from build123d import *

# Parameters (mm, degrees)
BOSS_EXTRUDE1_OUTLINE_R = 1.75
BOSS_EXTRUDE1_DEPTH     = 4
CUT_EXTRUDE1_DEPTH      = 1


# Read off the part's stored shape, not the designer's step: Boss-Extrude1
with BuildPart() as part:
    # Boss-Extrude1 outline → Boss-Extrude1 (new body)
    with BuildSketch(Plane(origin=(0, 0, 0), x_dir=(1, 0, 0), z_dir=(0, 1, 0))):
        with BuildLine():
            Line((25.086474615, -10.33744254), (36.25307775, -10.33744254))
            ThreePointArc((36.25307775, -10.33744254), (38.689776183, -5.587442326), (41.126474615, -10.33744254))
            Line((41.126474615, -10.33744254), (48.189776182, -10.33744254))
            Line((48.189776182, -10.33744254), (48.189776182, -18.81631662))
            Line((48.189776182, -18.81631662), (58.639776182, -18.81631662))
            Line((58.639776182, -18.81631662), (58.639776182, -4.977921711))
            Line((58.639776182, -4.977921711), (-21.360223818, -4.977921711))
            Line((-21.360223818, -4.977921711), (-21.360223818, -18.81631662))
            Line((-21.360223818, -18.81631662), (-10.910223818, -18.81631662))
            Line((-10.910223818, -18.81631662), (-10.910223818, -10.33744254))
            Line((-10.910223818, -10.33744254), (4.17307775, -10.33744254))
            ThreePointArc((4.17307775, -10.33744254), (6.609776182, -5.587442326), (9.046474615, -10.33744254))
            Line((9.046474615, -10.33744254), (20.21307775, -10.33744254))
            ThreePointArc((20.21307775, -10.33744254), (22.649776182, -5.587442326), (25.086474615, -10.33744254))
        make_face()
        with Locations((-16.360223818, -13.587442433)):
            Circle(BOSS_EXTRUDE1_OUTLINE_R, mode=Mode.SUBTRACT)
        with Locations((53.639776182, -13.587442433)):
            Circle(BOSS_EXTRUDE1_OUTLINE_R, mode=Mode.SUBTRACT)
    extrude(amount=BOSS_EXTRUDE1_DEPTH)

    # Sketch2 → Cut-Extrude1 (cut)
    # profile 1 of 2: a face of its own
    with BuildSketch(Plane(origin=(0, 4, 0), x_dir=(1, 0, 0), z_dir=(0, 1, 0))):
        Polygon((-16.41198232, -6.812466594), (-14.865187448, -6.812466594), (-14.865187448, -7.382338389), (-15.842110525, -7.382338389), (-15.842110525, -7.992915312), (-14.865187448, -7.992915312), (-14.865187448, -8.562787107), (-15.842110525, -8.562787107), (-15.842110525, -9.987466594), (-16.41198232, -9.987466594), align=None)
    # profile 2 of 2: a face of its own
    with BuildSketch(Plane(origin=(0, 4, 0), x_dir=(1, 0, 0), z_dir=(0, 1, 0))):
        with BuildLine():
            Line((-13.412523186, -6.731056337), (-12.907525189, -6.987371442))
            Line((-12.907525189, -6.987371442), (-13.460860525, -8.074325568))
            add(Edge.make_bspline(
                [(-13.460860525, -8.074325568), (-13.428168252, -8.075158914), (-13.363985411, -8.076794974), (-13.269480346, -8.090388716), (-13.179110672, -8.113598896), (-13.09179585, -8.144481034), (-13.008800475, -8.185943305), (-12.928789535, -8.235267944), (-12.853832504, -8.295423778), (-12.782210807, -8.362073474), (-12.717085558, -8.435911696), (-12.660512768, -8.515253227), (-12.611210579, -8.59816766), (-12.572885042, -8.686509995), (-12.541970388, -8.778815858), (-12.519664104, -8.875454234), (-12.506937745, -8.976704968), (-12.505183204, -9.045489177), (-12.504290013, -9.080505456)],
                knots=[0, 0, 0, 0, 1.013672955, 1.990085268, 2.953345895, 3.903887042, 4.856677135, 5.825509993, 6.813434118, 7.832212698, 8.85718992, 9.860832204, 10.8510077, 11.84312444, 12.841215551, 13.86684641, 14.914066156, 16, 16, 16, 16], degree=3))
            add(Edge.make_bspline(
                [(-12.504290013, -9.080505456), (-12.505127007, -9.114259025), (-12.506781387, -9.180975356), (-12.520457023, -9.278964679), (-12.54255757, -9.372979704), (-12.57414369, -9.462832672), (-12.614292202, -9.548962785), (-12.663391114, -9.631319503), (-12.721847604, -9.7092874), (-12.78815132, -9.782452193), (-12.860632718, -9.849142442), (-12.937032061, -9.908420617), (-13.017996745, -9.957386638), (-13.101996444, -9.998739592), (-13.190577642, -10.029597853), (-13.28241472, -10.052890494), (-13.378204103, -10.06633136), (-13.443223482, -10.068021564), (-13.476124948, -10.06887685)],
                knots=[0, 0, 0, 0, 1.049934834, 2.075270938, 3.072134561, 4.05064612, 5.033440221, 6.024524368, 7.028587226, 8.060776465, 9.092543989, 10.090062252, 11.064205434, 12.031961459, 12.998029633, 13.977230324, 14.976426867, 16, 16, 16, 16], degree=3))
            add(Edge.make_bspline(
                [(-13.476124948, -10.06887685), (-13.510529884, -10.068174962), (-13.578182536, -10.066794794), (-13.677175296, -10.051340548), (-13.772117873, -10.028076335), (-13.862476674, -9.994858992), (-13.948813614, -9.952563006), (-14.03011223, -9.900225978), (-14.107057351, -9.838425045), (-14.17882863, -9.768550629), (-14.243489203, -9.692012768), (-14.30116103, -9.61254654), (-14.349951471, -9.530027246), (-14.389446195, -9.444543116), (-14.420260894, -9.356366547), (-14.44170164, -9.265330188), (-14.455672265, -9.171675513), (-14.457310002, -9.108116151), (-14.458136166, -9.076053333)],
                knots=[0, 0, 0, 0, 1.063775006, 2.091769615, 3.092589432, 4.084662827, 5.064601646, 6.061867366, 7.070035304, 8.113879863, 9.156342271, 10.166834137, 11.149076039, 12.117706134, 13.076241869, 14.034148791, 15.008317125, 16, 16, 16, 16], degree=3))
            add(Edge.make_bspline(
                [(-14.458136166, -9.076053333), (-14.457699638, -9.05122443), (-14.45682415, -9.001428418), (-14.448026022, -8.926861595), (-14.434649776, -8.852099041), (-14.419144957, -8.789012031), (-14.40317966, -8.735665362), (-14.387110466, -8.690519517), (-14.367196241, -8.640417501), (-14.344431332, -8.585231374), (-14.318099865, -8.525027523), (-14.288339392, -8.45997005), (-14.255075822, -8.38956629), (-14.231354315, -8.341209808), (-14.218993538, -8.316012267)],
                knots=[0, 0, 0, 0, 1.110454016, 2.227089276, 3.35462975, 4.507227546, 5.131400587, 5.845402449, 6.650387134, 7.543487832, 8.516250726, 9.590168902, 10.744287919, 12, 12, 12, 12], degree=3))
            Line((-14.218993538, -8.316012267), (-13.412523186, -6.731056337))
        make_face()
        with BuildLine():
            add(Edge.make_bspline(
                [(-13.488845301, -8.603492235), (-13.516189484, -8.604746455), (-13.569698461, -8.607200799), (-13.645780224, -8.632903881), (-13.71514953, -8.67322562), (-13.775279703, -8.729381439), (-13.825573059, -8.796489848), (-13.862530382, -8.873035953), (-13.884762266, -8.957998267), (-13.887072017, -9.0174025), (-13.888264372, -9.048068557)],
                knots=[0, 0, 0, 0, 0.981744412, 1.921144944, 2.858899012, 3.85339082, 4.86292663, 5.863643845, 6.897155691, 8, 8, 8, 8], degree=3))
            add(Edge.make_bspline(
                [(-13.888264372, -9.048068557), (-13.886852586, -9.078744826), (-13.884106568, -9.138412221), (-13.861038737, -9.224183527), (-13.823269539, -9.302467905), (-13.770300647, -9.370465646), (-13.708115929, -9.426909036), (-13.639160453, -9.468651622), (-13.56458442, -9.494295462), (-13.512998357, -9.497424351), (-13.486937248, -9.499005055)],
                knots=[0, 0, 0, 0, 1.098279937, 2.136227893, 3.159405121, 4.194678092, 5.206500211, 6.154139736, 7.067477469, 8, 8, 8, 8], degree=3))
            add(Edge.make_bspline(
                [(-13.486937248, -9.499005055), (-13.459413771, -9.497396198), (-13.405435452, -9.494240948), (-13.327568188, -9.469676154), (-13.256435974, -9.428632893), (-13.193541338, -9.372370211), (-13.13951604, -9.305148416), (-13.102135992, -9.226404206), (-13.078001724, -9.140013833), (-13.075470478, -9.079404145), (-13.074161807, -9.048068557)],
                knots=[0, 0, 0, 0, 0.96921794, 1.900804717, 2.848419905, 3.844199796, 4.861108892, 5.867439427, 6.897452859, 8, 8, 8, 8], degree=3))
            add(Edge.make_bspline(
                [(-13.074161807, -9.048068557), (-13.075652622, -9.017420405), (-13.078539758, -8.95806668), (-13.100225571, -8.872706338), (-13.138944126, -8.79645527), (-13.19037541, -8.729104426), (-13.252574944, -8.672973647), (-13.324720551, -8.632585891), (-13.404277856, -8.607246336), (-13.460245153, -8.604761847), (-13.488845301, -8.603492235)],
                knots=[0, 0, 0, 0, 1.083229974, 2.097801324, 3.086792542, 4.086858909, 5.079819718, 6.026392613, 6.991456328, 8, 8, 8, 8], degree=3))
        make_face(mode=Mode.SUBTRACT)
    extrude(amount=-CUT_EXTRUDE1_DEPTH, mode=Mode.SUBTRACT)


solid = part.part
Design review of the part built by this model. Coordinates are the model's own, in mm. A direction names the side the tool comes from. Give positions to 0.01 mm unless a question says otherwise; leave off trailing zeros. Order: outer loops, then holes, each group sorted by start corner. A loop starts at its lowest first (then second) coordinate and runs counter-clockwise, first axis right, second up. Notation, with made-up numbers: (89, -29.5) - (101, -29.5) arc R24 cw to (101, 1.5) - close; hole circle Ø8 at (-3, -25.75). An arc over 180 degrees is marked (long way). Write item = value, one per line. Start each with the question number.
Q1. To check wall thickness, follow L1, parallel to X at y = 2.5, z = 7; L2, parallel to Z at x = -16, y = 3.35; L3, parallel to X at y = 0.6, z = 7.5. State the ranges of each line that lie inside material, in increasing order. Write a range as from..to.
Q2. We need section B-B on z = 14.25. State the section outline as (x, y) points.
Q3. We need section D-D on y = 0.65. State the section outline as (x, z) points.
Q4. Clearance check with a flat-ended pin moving along its axis: pin 1 Ø2 at (x, y) = (15.5, 2.5) entering from +Z. State where the tip first meets the part, or that it passes through.
Q5. Tool access review of faces 5 (the face through (15, 2, 10.337)), 6 (the face through (53, 2, 18.816)): name each direction out of +Z, -Z, +X, -X, +Y, -Y from which nothing blocks a thin tool from reaching the whole face with its end or side.
Q6. We need section A-A on z = 17.5. State the section outline as (x, y) points.
Q7. Mouldability with a two-part tool opening along Z and no side actions: class faces 1 (the face through (45, 2, 10.337)), 2 (the face through (6.52, 1.97, 5.59)), 3 (the face through (19, 2, 4.978)), 4 (the face through (-13.5, 3, 8.4)) as released by +Z, released by -Z, zero draft, split by the parting line, or undercut.
Q8. We need section C-C on x = 53.5. State the section outline as (y, z) points, plus the area to 3 significant figures.
Working result:
q1.L1 = -21.36..4.06, 9.16..20.1, 25.2..36.14, 41.24..58.64
q1.L2 = 4.98..6.81, 9.99..11.87, 15.3..18.82
q1.L3 = -21.36..3.81, 9.41..19.85, 25.45..35.89, 41.49..58.64
q2.outline = (-21.36, 0) - (-17.98, 0) - (-17.98, 4) - (-21.36, 4) - close; (-14.74, 0) - (-10.91, 0) - (-10.91, 4) - (-14.74, 4) - close; (48.19, 0) - (52.02, 0) - (52.02, 4) - (48.19, 4) - close; (55.26, 0) - (58.64, 0) - (58.64, 4) - (55.26, 4) - close
q3.outline = (-21.36, 4.98) - (58.64, 4.98) - (58.64, 18.82) - (48.19, 18.82) - (48.19, 10.34) - (41.13, 10.34) arc R3 cw (long way) to (36.25, 10.34) - (25.09, 10.34) arc R3 cw (long way) to (20.21, 10.34) - (9.05, 10.34) arc R3 cw (long way) to (4.17, 10.34) - (-10.91, 10.34) - (-10.91, 18.82) - (-21.36, 18.82) - close; hole circle Ø3.5 at (-16.36, 13.59); hole circle Ø3.5 at (53.64, 13.59)
q4.pin_1 = 10.34
q5.face_5 = +Z, +Y, -Y
q5.face_6 = +Z, +X, -X, +Y, -Y
q6.outline = (-21.36, 0) - (-10.91, 0) - (-10.91, 4) - (-21.36, 4) - close; (48.19, 0) - (58.64, 0) - (58.64, 4) - (48.19, 4) - close
q7.face_1 = released by +Z
q7.face_2 = undercut
q7.face_3 = released by -Z
q7.face_4 = undercut
q8.outline = (0, 4.98) - (4, 4.98) - (4, 11.84) - (0, 11.84) - close; (0, 15.33) - (4, 15.33) - (4, 18.82) - (0, 18.82) - close
q8.area = 41.4 mm²
